```python
from build123d import *

# Parameters (mm, degrees)
AUFSATZ_LINEAR_AUSTRAGEN1_DEPTH      = 35
SKIZZE3_R                            = 6
AUFSATZ_LINEAR_AUSTRAGEN2_DEPTH      = 5
SKIZZE4_R                            = 6.5
AUFSATZ_LINEAR_AUSTRAGEN3_DEPTH      = 0.1
SKIZZE7_R                            = 2.85
SCHNITT_LINEAR_AUSTRAGEN1_DEPTH      = 114.810889132
F_3_4_3_4_DURCHMESSER_BOHRUNG1_D     = 3.4
F_3_4_3_4_DURCHMESSER_BOHRUNG1_DEPTH = 4.5


with BuildPart() as part:
    # Skizze1 → Aufsatz-Linear austragen1 (new body)
    with BuildSketch(Plane(origin=(0, 0, 0), x_dir=(0, 0, -1), z_dir=(1, 0, 0))):
        Polygon((0, 0), (17.5, 0), (26.82, 0), (26.82, 118.310889132), (17.5, 118.310889132), (0, 88), align=None)
    extrude(amount=AUFSATZ_LINEAR_AUSTRAGEN1_DEPTH)

    # Skizze3 → Aufsatz-Linear austragen2 (add)
    with BuildSketch(Plane(origin=(0, 22, 38.105117767), x_dir=(1, 0, 0), z_dir=(0, 0.5, 0.866025404))):
        with Locations((17.5, 93.710235533)):
            Circle(SKIZZE3_R)
    extrude(amount=AUFSATZ_LINEAR_AUSTRAGEN2_DEPTH)

    # Skizze4 → Aufsatz-Linear austragen3 (add)
    with BuildSketch(Plane(origin=(0, 22, 38.105117767), x_dir=(1, 0, 0), z_dir=(0, 0.5, 0.866025404))):
        with Locations((17.5, 93.710235533)):
            Circle(SKIZZE4_R)
    extrude(amount=AUFSATZ_LINEAR_AUSTRAGEN3_DEPTH)

    # Skizze7 → Schnitt-Linear austragen1 (cut, through all)
    with BuildSketch(Plane(origin=(0, 4.5, 0), x_dir=(-1, 0, 0), z_dir=(0, -1, 0))):
        with Locations((-28.5, 5)):
            Circle(SKIZZE7_R)
        with Locations((-6.5, 5)):
            Circle(SKIZZE7_R)
        with Locations((-6.5, 21.82)):
            Circle(SKIZZE7_R)
        with Locations((-28.5, 21.82)):
            Circle(SKIZZE7_R)
    extrude(amount=-SCHNITT_LINEAR_AUSTRAGEN1_DEPTH, mode=Mode.SUBTRACT)

    # Ø3.4 (3.4) Durchmesser Bohrung1
    with Locations(Plane(origin=(6.5, 4.5, -5), x_dir=(0, 0, 1), z_dir=(0, 1, 0))):
        with Locations((0, 0), (-16.82, 0), (-16.82, 22), (0, 22)):
            Hole(F_3_4_3_4_DURCHMESSER_BOHRUNG1_D / 2, depth=F_3_4_3_4_DURCHMESSER_BOHRUNG1_DEPTH)


solid = part.part
```
Geometry check sheet. Reference: the model listing, model coordinates, mm. A direction names the side the tool comes from. Round coordinates to 2 decimals unless told otherwise and drop trailing zeros. Write each loop counter-clockwise with the first axis right and the second up, starting at its lowest first coordinate (ties: lowest second). Pieces come first, ordered by that corner, then holes. Notation, with made-up numbers: (-40, -34.75) -> (7, -34.75) arc R19 cw to (7, -8.75) -> close; hole circle Ø3 at (28, -27.5). An arc over 180 degrees is marked (long way). Put each result on its own line as item: value.
1) Access from +Z, -Z, +X, -X, +Y, -Y to the whole of each face (thin tool, end or side, straight path). Record for faces 1 (the face through (7, 4.5, -3)), 2 (the face through (0, 60, -13)).
Recorded:
face 1: +Y
face 2: +Z, -Z, -X, +Y, -Y
2) Cross-section at B-B, the plane z = -21.82. Enter the section's corners in (x, y).
Recorded:
outline: (0, 0) -> (4.8, 0) -> (4.8, 4.5) -> (3.65, 4.5) -> (3.65, 118.31) -> (0, 118.31) -> close; (8.2, 0) -> (26.8, 0) -> (26.8, 4.5) -> (25.65, 4.5) -> (25.65, 118.31) -> (9.35, 118.31) -> (9.35, 4.5) -> (8.2, 4.5) -> close; (30.2, 0) -> (35, 0) -> (35, 118.31) -> (31.35, 118.31) -> (31.35, 4.5) -> (30.2, 4.5) -> close
3) Cross-section at A-A, the plane y = 42. Enter the section's corners in (x, z), plus the area to 3 significant figures.
Recorded:
outline: (0, -26.82) -> (35, -26.82) -> (35, 0) -> (0, 0) -> close; hole circle Ø5.7 at (6.5, -21.82); hole circle Ø5.7 at (6.5, -5); hole circle Ø5.7 at (28.5, -21.82); hole circle Ø5.7 at (28.5, -5)
area: 837 mm2
4) Cross-section at D-D, the plane y = 93.5. Enter the section's corners in (x, z).
Recorded:
outline: (0, -26.82) -> (35, -26.82) -> (35, -3.18) -> (30.69, -3.18) arc R2.85 cw (long way) to (26.31, -3.18) -> (8.69, -3.18) arc R2.85 cw (long way) to (4.31, -3.18) -> (0, -3.18) -> close; hole circle Ø5.7 at (6.5, -21.82); hole circle Ø5.7 at (28.5, -21.82)
5) Depth check by flat-ended pin: P1, Ø2, axis at x = 13, z = -14.5, coming from the +Y side; P2, Ø12, axis at x = 14.5, z = -9, coming from the +Y side; P3, Ø2, axis at x = 6.5, z = -21.82, coming from the -Y side; P4, Ø6.5, axis at x = 6, z = -5.5, coming from the +Y side. Enter the tip coordinate at first touch or a pass-through.
Recorded:
P1: stops at y = 114.85
P2: stops at y = 113.98
P3: passes through
P4: stops at y = 103.16
6) Cross-section at C-C, the plane x = 28.5. Enter the section's corners in (y, z), plus the area to 3 significant figures.
Recorded:
outline: (0, -26.82) -> (118.31, -26.82) -> (118.31, -24.67) -> (4.5, -24.67) -> (4.5, -23.52) -> (0, -23.52) -> close; (0, -20.12) -> (4.5, -20.12) -> (4.5, -18.97) -> (118.31, -18.97) -> (118.31, -17.5) -> (101.6, -7.85) -> (4.5, -7.85) -> (4.5, -6.7) -> (0, -6.7) -> close; (0, -3.3) -> (4.5, -3.3) -> (4.5, -2.15) -> (91.72, -2.15) -> (88, 0) -> (0, 0) -> close
area: 1,700 mm2
7) Thickness scan on probe 1 along X at (y, z) = (3, -21.82); probe 2 along Z at (x, y) = (28.5, 30.5); probe 3 along X at (y, z) = (61.5, -5). Record the ranges inside material, lowest first. Write a range as from..to.
Recorded:
probe 1: x = 0..4.8, 8.2..26.8, 30.2..35
probe 2: z = -26.82..-24.67, -18.97..-7.85, -2.15..0
probe 3: x = 0..3.65, 9.35..25.65, 31.35..35
